Geometry check sheet. Reference: the model listing, model coordinates, mm. Give positions to 0.01 mm unless a question says otherwise; leave off trailing zeros. Order: outer loops, then holes, each group sorted by start corner. A loop starts at its lowest first (then second) coordinate and runs counter-clockwise, first axis right, second up. Notation, with made-up numbers: M 88.5,52.25 L 137.5,52.25 A17 cw 137.5,59.25 Z; hole C 18,44.5 d1. An arc over 180 degrees is marked long. Answer as CSV lines item,"result".
from build123d import *

# Parameters (mm, degrees)
SKETCH1_W           = 177.8
SKETCH1_H           = 177.8
SKETCH1_R           = 50.8
SKETCH1_R_2         = 3.175
SKETCH1_R_3         = 6.35
BOSS_EXTRUDE1_DEPTH = 25.4
FILLET1_R           = 6.35


with BuildPart() as part:
    # Sketch1 → Boss-Extrude1 (new body)
    with BuildSketch(Plane(origin=(0, 0, 0), x_dir=(1, 0, 0), z_dir=(0, 1, 0))):
        Rectangle(SKETCH1_W, SKETCH1_H)
        Circle(SKETCH1_R, mode=Mode.SUBTRACT)
        with Locations((44.45, 76.2)):
            Circle(SKETCH1_R_2, mode=Mode.SUBTRACT)
        with Locations((-44.45, 76.2)):
            Circle(SKETCH1_R_2, mode=Mode.SUBTRACT)
        with Locations((-76.2, 76.2)):
            Circle(SKETCH1_R_3, mode=Mode.SUBTRACT)
        with Locations((-76.2, -76.2)):
            Circle(SKETCH1_R_3, mode=Mode.SUBTRACT)
        with Locations((76.2, -76.2)):
            Circle(SKETCH1_R_3, mode=Mode.SUBTRACT)
        with Locations((76.2, 76.2)):
            Circle(SKETCH1_R_3, mode=Mode.SUBTRACT)
        with Locations((76.2, 44.45)):
            Circle(SKETCH1_R_2, mode=Mode.SUBTRACT)
        with Locations((76.2, -44.45)):
            Circle(SKETCH1_R_2, mode=Mode.SUBTRACT)
        with Locations((44.45, -76.2)):
            Circle(SKETCH1_R_2, mode=Mode.SUBTRACT)
        with Locations((-44.45, -76.2)):
            Circle(SKETCH1_R_2, mode=Mode.SUBTRACT)
        with Locations((-76.2, -44.45)):
            Circle(SKETCH1_R_2, mode=Mode.SUBTRACT)
        with Locations((-76.2, 44.45)):
            Circle(SKETCH1_R_2, mode=Mode.SUBTRACT)
    extrude(amount=BOSS_EXTRUDE1_DEPTH)

    # Fillet1
    fillet1_edges = [part.edges().sort_by_distance(p)[0] for p in [
        (-88.9, 12.7, -88.9),
        (88.9, 12.7, -88.9),
        (88.9, 12.7, 88.9),
        (-88.9, 12.7, 88.9),
    ]]
    fillet(fillet1_edges, radius=FILLET1_R)


solid = part.part
(1) Section check C-C on x = 0. Enter the section's corners in (y, z), then the cut area to 3 significant figures.
The answers:
outline,"M 0,-88.9 L 25.4,-88.9 L 25.4,-50.8 L 0,-50.8 Z; M 0,50.8 L 25.4,50.8 L 25.4,88.9 L 0,88.9 Z"
area,"1,940 mm2"
(2) Section check A-A on z = 76.2. Enter the section's corners in (x, y) (3 decimals).
The answers:
outline,"M -88.9,0 L -82.55,0 L -82.55,25.4 L -88.9,25.4 Z; M -69.85,0 L -47.625,0 L -47.625,25.4 L -69.85,25.4 Z; M -41.275,0 L 41.275,0 L 41.275,25.4 L -41.275,25.4 Z; M 47.625,0 L 69.85,0 L 69.85,25.4 L 47.625,25.4 Z; M 82.55,0 L 88.9,0 L 88.9,25.4 L 82.55,25.4 Z"
(3) Material ranges on line 1 (X direction, y = 12.5, z = -76.2) (3 decimals); line 2 (X direction, y = 16.5, z = 44.45) (3 decimals), recorded low to high.
The answers:
line 1,"x = -88.9 to -82.55, -69.85 to -47.625, -41.275 to 41.275, 47.625 to 69.85, 82.55 to 88.9"
line 2,"x = -88.9 to -79.375, -73.025 to -24.593, 24.593 to 73.025, 79.375 to 88.9"
(4) Draft check along Z on faces 1 (the face through (77.907, 12.522, -47.127)), 2 (the face through (-87.09, 12.88, 86.99)), 3 (the face through (38, 0, -41)). Enter one of: +Z half, -Z half, draft (parallel to the pull), parting line (faces both ways), or undercut.
The answers:
face 1,"undercut"
face 2,"+Z half"
face 3,"draft"
(5) Gauge pin test, flat end, axial feed: P1, Ø16.5, axis at x = 76.2, z = -76.2, coming from the -Y side. Record the tip position at first contact, or that the pin passes through.
The answers:
P1,"stops at y = 0"
(6) Section check D-D on z = -15. Enter the section's corners in (x, y), then the cut area to 3 significant figures.
The answers:
outline,"M -88.9,0 L -48.53,0 L -48.53,25.4 L -88.9,25.4 Z; M 48.53,0 L 88.9,0 L 88.9,25.4 L 48.53,25.4 Z"
area,"2,050 mm2"
(7) Section check B-B on y = 5. State how many separate pieces and enclosed holes the cut face has, then the cut area to 3 significant figures.
The answers:
separate pieces,"1"
enclosed holes,"13"
area,"22,700 mm2"
